from build123d import *

# Parameters (mm, degrees)
F0_R      = 12.1
F0_R_2    = 8.1
F1_DEPTH  = 6.4
F0_R_3    = 3.05
F0_W      = 5
F0_H      = 30
F2_DEPTH  = 3
F3_R      = 8.1
F3_R_2    = 7.1
F4_DEPTH  = 0.4
F5_DEPTH  = 35
F6_R      = 4.5
F7_DEPTH  = 10
F9_DEPTH  = 5
F11_DEPTH = 5
F12_W     = 35
F12_H     = 7.8
F12_R     = 3.05
F13_DEPTH = 1
F14_DEPTH = 46.301


with BuildPart() as f1:
    # F0 (on Front) → F1 (new body)
    with BuildSketch(Plane.XZ):
        Circle(F0_R)
        Circle(F0_R_2, mode=Mode.SUBTRACT)
    extrude(amount=F1_DEPTH)

    # F0 (on Front) → F2 (join)
    with BuildSketch(Plane.XZ):
        with BuildLine():
            Line((-21.65, 0.5412544591), (-21.65, -0.5412544591))
            ThreePointArc((-21.65, -0.5412544591), (-21.0942775075, -2.8321925717), (-19.5506410256, -4.6138803491))
            Line((-19.5506410256, -4.6138803491), (-6.2701517693, -14.0726258901))
            ThreePointArc((-6.2701517693, -14.0726258901), (-4.892151632, -14.7625166378), (-3.3695107437, -15))
            Line((-3.3695107437, -15), (19.65, -15))
            Line((19.65, -15), (19.65, 15))
            Line((19.65, 15), (-3.3695107437, 15))
            ThreePointArc((-3.3695107437, 15), (-4.892151632, 14.7625166378), (-6.2701517693, 14.0726258901))
            Line((-6.2701517693, 14.0726258901), (-19.5506410256, 4.6138803491))
            ThreePointArc((-19.5506410256, 4.6138803491), (-21.0942775075, 2.8321925717), (-21.65, 0.5412544591))
        make_face()
        with Locations((-15.6, 0)):
            Circle(F0_R_3, mode=Mode.SUBTRACT)
        Circle(F0_R, mode=Mode.SUBTRACT)
        with Locations((15.6, 0)):
            Circle(F0_R_3, mode=Mode.SUBTRACT)
        with Locations((22.15, 0)):
            Rectangle(F0_W, F0_H)
    extrude(amount=F2_DEPTH)

    # F3 (on face) → F4 (join)
    with BuildSketch(Plane(origin=(0, 0, 0), x_dir=(-1, 0, 0), z_dir=(0, 1, 0))):
        Circle(F3_R)
        Circle(F3_R_2, mode=Mode.SUBTRACT)
    extrude(amount=-F4_DEPTH)

    # F0 (on Front) → F5 (join)
    with BuildSketch(Plane.XZ):
        with Locations((22.15, 0)):
            Rectangle(F0_W, F0_H)
    extrude(amount=F5_DEPTH)

    # F6 (on face) → F7 (cut)
    with BuildSketch(Plane.XZ.offset(3)):
        with Locations((-15.6, 0)):
            Circle(F6_R)
        with Locations((15.6, 0)):
            Circle(F6_R)
    extrude(amount=F7_DEPTH, mode=Mode.SUBTRACT)

    # F8 (on face) → F9 (join)
    with BuildSketch(Plane(origin=(0, 0, -15), x_dir=(1, 0, 0), z_dir=(0, 0, -1))):
        Polygon((19.65, 3), (19.65, 35), (-3.3695107437, 3), align=None)
    extrude(amount=-F9_DEPTH)

    # F10 (on face) → F11 (join)
    with BuildSketch(Plane.XY.offset(15)):
        Polygon((19.65, -3), (-3.3695107437, -3), (19.65, -35), align=None)
    extrude(amount=-F11_DEPTH)

    # F12 (on face) → F13 (join)
    with BuildSketch(Plane.YZ.offset(24.65)):
        with Locations((-17.5, 0)):
            Rectangle(F12_W, F12_H)
        with Locations((-17.5, 0)):
            Circle(F12_R, mode=Mode.SUBTRACT)
    extrude(amount=F13_DEPTH)

    # F14 (cut, through all): a face of the model
    f14_faces = [f1.faces().sort_by_distance(p)[0] for p in [
        (24.65, -17.5, 0),
    ]]
    extrude(f14_faces, amount=-F14_DEPTH, mode=Mode.SUBTRACT)


solid = f1.part
Build history of the part. All positions in model axes, mm. A direction names the side the tool comes from. Round coordinates to 2 decimals unless told otherwise and drop trailing zeros. Order: outer loops, then holes, each group sorted by start corner. A loop starts at its lowest first (then second) coordinate and runs counter-clockwise, first axis right, second up. Notation, with made-up numbers: M -9.5,-31.75 L 11.5,-31.75 A19 ccw 11.5,-11.75 Z; hole C 7.5,32.25 d11. An arc over 180 degrees is marked long. Use CSV: the item, a comma, the result in double quotes. Start each with the question number.
(1) Cut at B-B on z = 0. State how many separate pieces and enclosed holes the cut face has, then the cut area to 3 significant figures.
(2) Cut at A-A on x = 15.6. List the corners of the cut face in (y, z), then the cut area to 3 significant figures.
(3) Flat gauge pins, fed straight in: P1, Ø0.5, axis at x = 25, y = -21.5, coming from the +Z side; P2, Ø3.5, axis at y = -16, z = -10.5, coming from the +X side; P3, Ø4, axis at x = 15, z = 3.5, coming from the -Y side; P4, Ø5.5, axis at y = -17.5, z = 0, coming from the -X side. Where does each tip first touch, or does it go through?
(4) Tool access for faces 5 (the face through (-11.1, -4.7, 0)), 6 (the face through (11.1, -4.7, 0)), 7 (the face through (24.65, -17, -10)): list every direction of +Z, -Z, +X, -X, +Y, -Y with a clear straight run to the whole face (end or side of a thin tool).
(5) Mould opens along Z. For faces 1 (the face through (-8, -6.4, -3)), 2 (the face through (0.92, -0.2, 7.04)), 3 (the face through (-21.65, -1, 0)), 4 (the face through (14, -14, -15)) say: +Z half, -Z half, draft (parallel to the pull), parting line (faces both ways), or undercut.
(6) Drill centre lines: probe 1 along Y at (x, z) = (20, -0.25); probe 2 along Z at (x, y) = (16.5, -14); probe 3 along Z at (x, y) = (0, -4). Where is each one in solid material? Low to high.
(7) Cut at D-D on y = -17.5. List the corners of the cut face in (x, z).
(8) Cut at C-C on y = -5.5. List the corners of the cut face in (x, z), then the cut area to 3 significant figures.
Findings:
1,separate pieces,"5"
1,enclosed holes,"0"
1,area,"229 mm^2"
2,outline,"M -29.37,-15 L 0,-15 L 0,-3.05 L -3,-3.05 L -3,-10 L -29.37,-10 Z; M -29.37,10 L -3,10 L -3,3.05 L 0,3.05 L 0,15 L -29.37,15 Z"
2,area,"335 mm^2"
3,P1,"stops at z = 3.9"
3,P2,"stops at x = 24.65"
3,P3,"stops at y = -3"
3,P4,"passes through"
4,face 5,"-X, -Y"
4,face 6,"-Y"
4,face 7,"-Z, +X, +Y, -Y"
5,face 1,"undercut"
5,face 2,"undercut"
5,face 3,"draft"
5,face 4,"-Z half"
6,probe 1,"y = -35 to -20.54, -14.46 to -13, -3 to 0"
6,probe 2,"z = -15 to -10, 10 to 15"
6,probe 3,"z = -15 to -8.1, 8.1 to 15"
7,outline,"M 7.06,-15 L 24.65,-15 L 24.65,-3.9 L 25.65,-3.9 L 25.65,-3.05 L 19.65,-3.05 L 19.65,-10 L 7.06,-10 Z; M 7.06,10 L 19.65,10 L 19.65,3.05 L 25.65,3.05 L 25.65,3.9 L 24.65,3.9 L 24.65,15 L 7.06,15 Z"
8,outline,"M -11.84,-2.48 A12.1 ccw -1.57,-12 L -1.57,-15 L 24.65,-15 L 24.65,-3.9 L 25.65,-3.9 L 25.65,3.9 L 24.65,3.9 L 24.65,15 L -1.57,15 L -1.57,12 A12.1 ccw -11.84,2.48 A4.5 cw Z; hole C 0,0 d16.2; hole M 6.81,-10 L 19.65,-10 L 19.65,-1.96 A4.5 ccw 19.65,1.96 L 19.65,10 L 6.81,10 A12.1 cw 11.84,2.48 A4.5 ccw 11.84,-2.48 A12.1 cw Z"
8,area,"590 mm^2"
